Read the model definition and answer for the solid it produces. Units are mm, in the model's axes. A direction names the side the tool comes from. Give positions to 0.01 mm unless a question says otherwise; leave off trailing zeros. Order: outer loops, then holes, each group sorted by start corner. A loop starts at its lowest first (then second) coordinate and runs counter-clockwise, first axis right, second up. Notation, with made-up numbers: (-2.75, 86.5) -> (15.25, 86.5) arc R16 ccw to (15.25, 100.5) -> close; hole circle Ø7 at (-14, 55.5). An arc over 180 degrees is marked (long way). Answer as CSV lines item,"result". Start each with the question number.
1) Flat-ended cylindrical pins translate along their axes: pin 1 Ø2 at (x, y) = (6.5, -18.5) entering from +Z; pin 2 Ø2 at (x, z) = (19.5, 1322.5) entering from -Y; pin 3 Ø6 at (y, z) = (-77, 1445.5) entering from -X. Find the tip coordinate at first contact, or state that the pin passes through.
2) For faces 4 (the face through (-45, 69.4, 1045)), 5 (the face through (0, -6, 2110)), 6 (the face through (1, 80.9, 1045)), 7 (the face through (45, -69.4, 1045)), 8 (the face through (-2, 2, 0)), determine the directions among +Z, -Z, +X, -X, +Y, -Y from which every point of the face is accessible in a straight line to the end or side of a thin tool.
3) The mould has two halves that part along X. Classify faces 1 (the face through (4, -1, 1045)), 2 (the face through (-4, 1, 1045)), 3 (the face through (-1, -80.9, 1045)): +X half, -X half, draft (parallel to the pull), parting line (faces both ways), or undercut.
4) Find section B-B (x = -129). Determine the outline of the cut face in (y, z), and give its area (3 significant figures).
5) Straight lines are drawn through the part: L1, parallel to Y at x = -75.5, z = 98.5; L2, parallel to Z at x = 81.5, y = -102.5; L3, parallel to X at y = -26, z = 1571. For each, find the intervals that lie inside material, in ascending order. Write a range as from..to.
6) Find section A-A (z = 858). Determine the outline of the cut face in (x, y), and give its area (3 significant figures).
```python
from build123d import *

# Parameters (mm, degrees)
F0_W     = 300
F0_H     = 300
F1_DEPTH = 10
F3_DEPTH = 2100


with BuildPart() as f1:
    # F0 (on Top) → F1 (new body)
    with BuildSketch(Plane.XY):
        Rectangle(F0_W, F0_H)
    extrude(amount=F1_DEPTH)

    # F2 (on face) → F3 (join)
    with BuildSketch(Plane.XY.offset(10)):
        with BuildLine():
            Line((77.2, 80.9), (-77.2, 80.9))
            Line((-77.2, 80.9), (-77.2, 69.4))
            Line((-77.2, 69.4), (-11.6, 69.4))
            ThreePointArc((-11.6, 69.4), (-6.225988, 67.174012), (-4, 61.8))
            Line((-4, 61.8), (-4, -61.8))
            ThreePointArc((-4, -61.8), (-6.225988, -67.174012), (-11.6, -69.4))
            Line((-11.6, -69.4), (-77.2, -69.4))
            Line((-77.2, -69.4), (-77.2, -80.9))
            Line((-77.2, -80.9), (77.2, -80.9))
            Line((77.2, -80.9), (77.2, -69.4))
            Line((77.2, -69.4), (11.6, -69.4))
            ThreePointArc((11.6, -69.4), (6.225988, -67.174012), (4, -61.8))
            Line((4, -61.8), (4, 61.8))
            ThreePointArc((4, 61.8), (6.225988, 67.174012), (11.6, 69.4))
            Line((11.6, 69.4), (77.2, 69.4))
            Line((77.2, 69.4), (77.2, 80.9))
        make_face()
    extrude(amount=F3_DEPTH)


solid = f1.part
```
Findings below:
1,pin 1,"z = 10"
1,pin 2,"y = -80.9"
1,pin 3,"x = -77.2"
2,face 4,"+Z, -X"
2,face 5,"+Z, +X, -X, +Y, -Y"
2,face 6,"+Z, +X, -X, +Y"
2,face 7,"+Z, +X"
2,face 8,"-Z, +X, -X, +Y, -Y"
3,face 1,"+X half"
3,face 2,"-X half"
3,face 3,"draft"
4,outline,"(-150, 0) -> (150, 0) -> (150, 10) -> (-150, 10) -> close"
4,area,"3,000 mm²"
5,L1,"-80.9..-69.4, 69.4..80.9"
5,L2,"0..10"
5,L3,"-4..4"
6,outline,"(-77.2, -80.9) -> (77.2, -80.9) -> (77.2, -69.4) -> (11.6, -69.4) arc R7.6 cw to (4, -61.8) -> (4, 61.8) arc R7.6 cw to (11.6, 69.4) -> (77.2, 69.4) -> (77.2, 80.9) -> (-77.2, 80.9) -> (-77.2, 69.4) -> (-11.6, 69.4) arc R7.6 cw to (-4, 61.8) -> (-4, -61.8) arc R7.6 cw to (-11.6, -69.4) -> (-77.2, -69.4) -> close"
6,area,"4,710 mm²"
